Check sheet for the modelled part. Datum: model origin and axes. Units: mm. A direction names the side the tool comes from. Coordinates: 2 decimals unless noted, no trailing zeros. Write each loop counter-clockwise with the first axis right and the second up, starting at its lowest first coordinate (ties: lowest second). Pieces come first, ordered by that corner, then holes. Notation, with made-up numbers: (-14.5, 3.25) - (7.5, 3.25) arc R8 ccw to (7.5, 14.25) - close; hole circle Ø8 at (-2.75, -37.75). An arc over 180 degrees is marked (long way). Use one line per item in the form item = value. Start each with the question number.
1. Tool access check on faces 4 (the face through (2, -3, 0)), 5 (the face through (-2, -2, -6.35)), 6 (the face through (0, -2.381, -5)). Record the directions out of +Z, -Z, +X, -X, +Y, -Y that give a thin tool (end or side, any length) a straight path to the whole face; none if there is none.
2. Cross-section at A-A on z = 44.5. Record the boundary of the cut face in (x, y) (3 decimals), then the cut area to 3 significant figures.
3. Draft check along Y on faces 1 (the face through (-0.69, 3.1, 31.06)), 2 (the face through (0, 0, -3.175)), 3 (the face through (0, 0, 63.5)). Enter one of: +Y half, -Y half, draft (parallel to the pull), parting line (faces both ways), or undercut.
4. Go/stop test with flat-tipped pins: pin 1 Ø2 at (x, y) = (1.5, -3.5) entering from +Z; pin 2 Ø5 at (x, y) = (-0.5, 0) entering from -Z; pin 3 Ø3 at (x, z) = (1, 50.5) entering from +Y (3 decimals); pin 4 Ø4 at (y, z) = (-2.5, 49) entering from -X. Record where each tip stops, or that it passes through.
5. Scan lines: line 1 along Z through (x, y) = (-0.75, 1) (3 decimals); line 2 along Z through (x, y) = (-0.5, -3.75); line 3 along Y through (x, z) = (-1, 2.5). Record each from-to range of solid material in increasing order.
Autodesk Inventor part; units mm, degrees
ref_plane "YZ Plane" through (0, 0, 0) normal (1, 0, 0) x (0, 1, 0)
ref_plane "XZ Plane" through (0, 0, 0) normal (0, 1, 0) x (-1, 0, 0)
ref_plane "XY Plane" through (0, 0, 0) normal (0, 0, 1) x (1, 0, 0)
sketch "Sketch1" plane through (0, 0, 0) normal (0, 0, 1) x (1, 0, 0)
  circle A0 centre (0, 0) radius 3.175
  dimension "d0" = 6.35
extrude "Extrusion1" add sketch "Sketch1" along normal blind 63.5
sketch "Sketch2" plane through (0, 0, 0) normal (0, 0, -1) x (-1, 0, 0)
  circle A0 centre (0, 0) radius 3.175
  circle A1 centre (0, 0) radius 4.7625
  dimension "d3" = 9.525
extrude "Extrusion2" add sketch "Sketch2" along normal blind 6.35 contours A0 | A1
sketch "Sketch3" plane through (0, 0, -6.35) normal (0, 0, -1) x (-1, 0, 0)
  circle A0 centre (0, 0) radius 4.7625
  line L0 (-1.3748, 2.3812) -> (1.3748, 2.3813)
  line L1 (1.3748, 2.3813) -> (2.7496, 0)
  line L2 (2.7496, 0) -> (1.3748, -2.3812)
  line L3 (1.3748, -2.3812) -> (-1.3748, -2.3812)
  line L4 (-1.3748, -2.3812) -> (-2.7496, 0)
  line L5 (-2.7496, 0) -> (-1.3748, 2.3812)
  dimension "d6" = 4.7625
extrude "Extrusion3" cut sketch "Sketch3" against normal blind 3.175 contours L0 L1 L2 L3 L4 L5
chamfer "Chamfer1" distance 0.508 angle 45 3 edges at (-3.175, 0, 63.5) (4.7625, 0, 0) (4.7625, 0, -6.35)
thread "Thread1"
properties part number "14-20 x2500" material "Steel"
Final values:
q1.face_4 = +Z
q1.face_5 = -Z, +X, -X, +Y, -Y
q1.face_6 = -Z
q2.outline = circle Ø6.35 at (0, 0)
q2.area = 31.7 mm²
q3.face_1 = parting line
q3.face_2 = undercut
q3.face_3 = draft
q4.pin_1 = 63.36
q4.pin_2 = -6.35
q4.pin_3 = 3.175
q4.pin_4 = -3.14
q5.line_1 = -3.175 to 63.5
q5.line_2 = -6.35 to 0
q5.line_3 = -3.01 to 3.01
